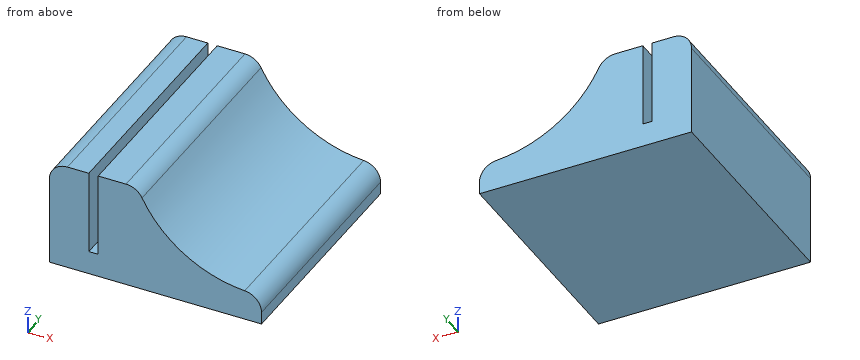
```python
from build123d import *

# Parameters (mm, degrees)
F1_DEPTH = 64
F2_W     = 2.6
F2_H     = 64
F3_DEPTH = 23.4
F4_R     = 5


with BuildPart() as f1:
    # F0 (on Front) → F1 (new body)
    with BuildSketch(Plane.XZ):
        with BuildLine():
            Line((24.4545675814, -5.1988300681), (0, -5.1988300681))
            Line((0, -5.1988300681), (0, -35.1988300681))
            Line((0, -35.1988300681), (58.8754676282, -35.1988300681))
            Line((58.8754676282, -35.1988300681), (58.8754676282, -26.7230011523))
            ThreePointArc((58.8754676282, -26.7230011523), (38.1790837444, -21.5355312603), (24.4545675814, -5.1988300681))
        make_face()
    extrude(amount=F1_DEPTH)

    # F2 (on face) → F3 (cut)
    with BuildSketch(Plane.XY.offset(-5.1988300681)):
        with Locations((12.2272837907, -32)):
            Rectangle(F2_W, F2_H)
    extrude(amount=-F3_DEPTH, mode=Mode.SUBTRACT)

    # F4
    f4_edges = [f1.edges().sort_by_distance(p)[0] for p in [
        (24.454568, -32, -5.19883),
        (0, -32, -5.19883),
        (58.875468, -32, -26.723001),
    ]]
    fillet(f4_edges, radius=F4_R)


solid = f1.part
```
Input: part model. Units: mm. Frame: model coordinates. Give positions to 0.01 mm unless a question says otherwise; leave off trailing zeros. Order: outer loops, then holes, each group sorted by start corner. A loop starts at its lowest first (then second) coordinate and runs counter-clockwise, first axis right, second up. Notation, with made-up numbers: (19, 11.25) -> (41, 11.25) arc R26 cw to (41, 25.25) -> close; hole circle Ø6 at (49.5, 15.25). An arc over 180 degrees is marked (long way). Write each question's results on one line, items separated by ' | '. Start each with the question number.
Item 1: Cut plane C-C on x = 12. Return the cut outline in (y, z).
Item 2: Cut plane A-A on z = -21. Return the cut outline in (x, y), then the cut area to 3 significant figures.
Item 3: Cut plane B-B on y = -56. Return the cut outline in (x, z), then the cut area to 3 significant figures.
Item 4: Line query: line 1 (X direction, y = -55, z = -19.25); line 2 (X direction, y = -41.5, z = -12.25); line 3 (Z direction, x = 12, y = -10). Output: solid intervals per line, ascending.
Item 5: Contact query for flat-ended pins moving along their axis: P1, Ø4, axis at x = 48.5, y = -20, coming from the +Z side; P2, Ø2, axis at x = 12, y = -45.5, coming from the +Z side; P3, Ø2, axis at y = -33, z = -22.5, coming from the +X side. Output: stop coordinate, or through.
Item 6: Cut plane D-D on z = -15.25. Return the cut outline in (x, y).
Established:
1) outline: (-64, -35.2) -> (0, -35.2) -> (0, -28.6) -> (-64, -28.6) -> close
2) outline: (0, -64) -> (10.93, -64) -> (10.93, 0) -> (0, 0) -> close; (13.53, -64) -> (37.35, -64) -> (37.35, 0) -> (13.53, 0) -> close | area: 2,220 mm^2
3) outline: (0, -35.2) -> (58.88, -35.2) -> (58.88, -31.71) arc R5 ccw to (54.21, -26.72) arc R34.62 cw to (25.7, -7.93) arc R5 ccw to (21.25, -5.2) -> (13.53, -5.2) -> (13.53, -28.6) -> (10.93, -28.6) -> (10.93, -5.2) -> (5, -5.2) arc R5 ccw to (0, -10.2) -> close | area: 1,140 mm^2
4) line 1: 0 to 10.93, 13.53 to 34.95 | line 2: 0 to 10.93, 13.53 to 28.32 | line 3: -35.2 to -28.6
5) P1: z = -25.32 | P2: z = -28.6 | P3: x = 41.78
6) outline: (0, -64) -> (10.93, -64) -> (10.93, 0) -> (0, 0) -> close; (13.53, -64) -> (30.72, -64) -> (30.72, 0) -> (13.53, 0) -> close
